Geometry: final body of the model. Coordinates: model frame, mm. Face numbers are marked on the shaded views. A direction names the side the tool comes from. Give positions to 0.01 mm unless a question says otherwise; leave off trailing zeros. Loops run counter-clockwise (first coordinate to the right, second up) from the corner with the lowest first, then second, coordinate; pieces in that order, holes last. Notation, with made-up numbers: M 39.25,-22 L 69.25,-22 A13 cw 69.25,0 Z; hole C 59.25,34 d8. An arc over 180 degrees is marked long. One line per question, with ' | ' between items. Start each with the question number.
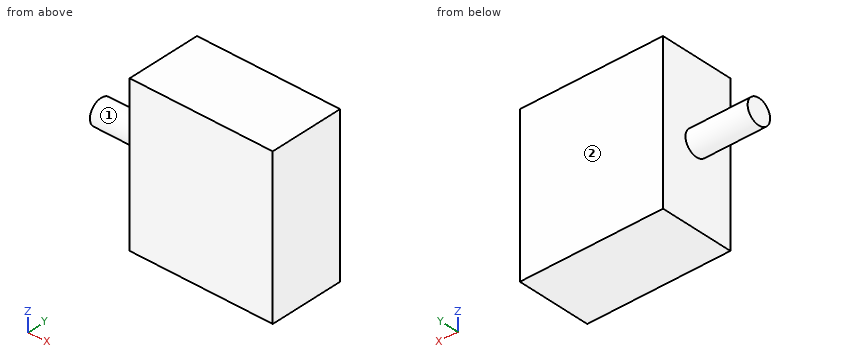
from build123d import *

# Parameters (mm, degrees)
ESQUISSE1_W        = 23
ESQUISSE1_H        = 12
BOSS_EXTRU_1_DEPTH = 25
ESQUISSE4_R        = 2
BOSS_EXTRU_2_DEPTH = 10


with BuildPart() as part:
    # Esquisse1 → Boss.-Extru.1 (new body)
    with BuildSketch(Plane.XY):
        with Locations((11.5, 6)):
            Rectangle(ESQUISSE1_W, ESQUISSE1_H)
    extrude(amount=BOSS_EXTRU_1_DEPTH)

    # Esquisse4 → Boss.-Extru.2 (add)
    with BuildSketch(Plane.ZY):
        with Locations(Location((12.5, 6, 0), (0, 0, 180))):
            Circle(ESQUISSE4_R)
    extrude(amount=BOSS_EXTRU_2_DEPTH)


solid = part.part
Q1. Material intervals for L1, parallel to X at y = 6, z = 3.5; L2, parallel to Z at x = -2, y = 6, sorted ascending.
Q2. Set-up query: the marked faces 1 and 2. Return all of +Z, -Z, +X, -X, +Y, -Y with unobstructed straight access to the full face (end or side cutting, diameter ignored); none if empty.
Q3. Section A-A, the plane y = 6. Output: boundary loops of the cut face in (x, z), plus the area to 3 significant figures.
Q4. Contact query for flat-ended pins moving along their axis: pin 1 (4 mm diameter, centred on y = 7, z = 6.5, fed in from -X); pin 2 (6 mm diameter, centred on x = -3.5, y = 4, fed in from +Z). Output: stop coordinate, or through.
Q5. Section C-C, the plane x = -5. Output: boundary loops of the cut face in (y, z).
Q6. Section D-D, the plane y = 10.75. Output: boundary loops of the cut face in (x, z).
Q7. Section B-B, the plane z = 12.5. Output: boundary loops of the cut face in (x, y), plus the area to 3 significant figures.
Model answer:
1) L1: x = 0 to 23 | L2: z = 10.5 to 14.5
2) face 1: -X | face 2: +Z, -Z, +X, -X, +Y
3) outline: M -10,10.5 L 0,10.5 L 0,0 L 23,0 L 23,25 L 0,25 L 0,14.5 L -10,14.5 Z | area: 615 mm^2
4) pin 1: stops at x = 0 | pin 2: stops at z = 14.5
5) outline: C 6,12.5 d4
6) outline: M 0,0 L 23,0 L 23,25 L 0,25 Z
7) outline: M -10,4 L 0,4 L 0,0 L 23,0 L 23,12 L 0,12 L 0,8 L -10,8 Z | area: 316 mm^2
